Input: part model. Units: mm. Frame: model coordinates. A direction names the side the tool comes from. Coordinates: 2 decimals unless noted, no trailing zeros. Order: outer loops, then holes, each group sorted by start corner. A loop starts at its lowest first (then second) coordinate and runs counter-clockwise, first axis right, second up. Notation, with made-up numbers: (63, -19.75) -> (100, -19.75) arc R21 ccw to (100, 17.25) -> close; hole circle Ø3 at (73, 59). An arc over 180 degrees is marked (long way). Use CSV: the item, a comma, the result in double quotes. Start each with the question number.
Autodesk Inventor part; units mm, degrees
ref_plane "Work Plane1" through (0, 1.5, 0) normal (0, 1, 0) x (1, 0, 0)
ref_plane "YZ Plane" through (0, 0, 0) normal (1, 0, 0) x (0, 1, 0)
ref_plane "XZ Plane" through (0, 0, 0) normal (0, 1, 0) x (-1, 0, 0)
sketch "Sketch1" plane through (0, 0, 0) normal (0, 1, 0) x (-1, 0, 0)
  circle A0 centre (0, 0) radius 8.825
  dimension "d0" = 17.65
extrude "Extrusion1" add sketch "Sketch1" along normal blind 3
sketch "Sketch2" plane through (0, 0, 0) normal (0, -1, 0) x (1, 0, 0)
  circle A0 centre (0, 0) radius 8.825
  circle A1 centre (0, 0) radius 2.75
  dimension "d3" = 5.5
extrude "Extrusion2" add sketch "Sketch2" along normal blind 5 contours A1
sketch "Sketch3" plane through (0, 3, 0) normal (0, 1, 0) x (1, 0, 0)
  circle A0 centre (0, 0) radius 8.825
  circle A1 centre (-6, 0) radius 2
  line L0 (-6, 0) -> (5.0545, 0) construction
  circle A2 centre (0, -6) radius 2
  circle A3 centre (6, 0) radius 2
  circle A4 centre (0, 6) radius 2
  circle A5 centre (-4.2426, 4.2426) radius 0.8
  line L1 (0, 0) -> (-4.2426, 4.2426) construction
  circle A6 centre (0, 0) radius 2.75
  arc A7 (0, 6) -> (-6, 0) centre (0, 0) ccw construction
  circle A8 centre (-4.2426, -4.2426) radius 0.8
  circle A9 centre (4.2426, -4.2426) radius 0.8
  circle A10 centre (4.2426, 4.2426) radius 0.8
  dimension "d6" = 4
  dimension "d7" = 6
  dimension "d10" = 360
  dimension "d14" = 1.6
  dimension "d15" = 45
  dimension "d18" = 360
extrude "Extrusion3" cut sketch "Sketch3" against normal through all contours A1 | A2 | A3 | A4 | A5 | A8 | A9 | A10
sketch "Sketch4" plane through (0, 3, 0) normal (0, 1, 0) x (1, 0, 0)
  circle A0 centre (6, 0) radius 2
  circle A1 centre (-6, 0) radius 2
  circle A2 centre (0, -6) radius 2
  circle A3 centre (0, 6) radius 2
  circle A4 centre (0, 6) radius 2.4
  circle A5 centre (-6, 0) radius 2.4
  circle A6 centre (6, 0) radius 2.4
  circle A7 centre (0, -6) radius 2.4
  dimension "d20" = 0.4
  dimension "d21" = 0.4
  dimension "d22" = 0.4
  dimension "d23" = 0.4
extrude "Extrusion4" cut sketch "Sketch4" against normal blind 0.8
ref_plane "Work Plane1" through (0, 1.5, 0) normal (0, 1, 0) x (1, 0, 0)
mirror "Mirror1" about plane through (0, 1.5, 0) normal (0, 1, 0) of "Extrusion4"
properties part number "xl320_wheel" material "PC/ABS Plastic"
1. Section C-C on x = 6. Return loops of the section in (y, z), then the cut area to 3 significant figures.
2. Contact query for flat-ended pins moving along their axis: P1, Ø1.4, axis at x = 4.24, z = 4.24, coming from the -Y side; P2, Ø2.5, axis at x = -4.24, z = 4.24, coming from the +Y side; P3, Ø5.5, axis at x = 0, z = -7, coming from the -Y side. Output: stop coordinate, or through.
3. Section A-A on z = 0. State how many separate pieces and enclosed holes the cut face has, then the cut area to 3 significant figures.
4. Material intervals for line 1 along Z through (x, y) = (0, 0.55) (3 decimals); line 2 along Z through (x, y) = (-4, 0.25); line 3 along Z through (x, y) = (0.5, 0.25), sorted ascending.
5. Access query for faces 5 (the face through (7, 0.8, -2)), 6 (the face through (-7.6, 1.5, 1.2)), 7 (the face through (-1, 2.2, 4)). Directions: +Z, -Z, +X, -X, +Y, -Y. A direction counts if a zero-diameter tool reaches every point of the face in a straight line with its end or side. Return the directions, or none.
6. Section D-D on y = -1.25. Return loops of the section in (x, z).
7. Pull-direction query (Z, two-part tool) for faces 1 (the face through (0, -5, 0)), 2 (the face through (-0.596, -2.465, 2.685)), 3 (the face through (1.29, 2.606, -8.024)), 4 (the face through (-7, 2.2, -2)); classes: released by +Z, released by -Z, zero draft, split by the parting line, or undercut.
8. Section B-B on z = -7. Return loops of the section in (x, y).
Values follow:
1,outline,"(0, -6.47) -> (3, -6.47) -> (3, -2.4) -> (2.2, -2.4) -> (2.2, -2) -> (0.8, -2) -> (0.8, -2.4) -> (0, -2.4) -> close; (0, 2.4) -> (0.8, 2.4) -> (0.8, 2) -> (2.2, 2) -> (2.2, 2.4) -> (3, 2.4) -> (3, 6.47) -> (0, 6.47) -> close"
1,area,"25.5 mm2"
2,P1,"passes through"
2,P2,"stops at y = 3"
2,P3,"stops at y = 0"
3,separate pieces,"3"
3,enclosed holes,"0"
3,area,"53.9 mm2"
4,line 1,"z = -8.825 to -8.4, -3.6 to 3.6, 8.4 to 8.825"
4,line 2,"z = -7.87 to -5, -3.48 to -1.33, 1.33 to 3.48, 5 to 7.87"
4,line 3,"z = -8.81 to -8.35, -3.65 to 3.65, 8.35 to 8.81"
5,face 5,"-Y"
5,face 6,"+Y, -Y"
5,face 7,"+Y"
6,outline,"circle Ø5.5 at (0, 0)"
7,face 1,"zero draft"
7,face 2,"split by the parting line"
7,face 3,"undercut"
7,face 4,"undercut"
8,outline,"(-5.37, 0) -> (-2.18, 0) -> (-2.18, 0.8) -> (-1.73, 0.8) -> (-1.73, 2.2) -> (-2.18, 2.2) -> (-2.18, 3) -> (-5.37, 3) -> close; (1.73, 0.8) -> (2.18, 0.8) -> (2.18, 0) -> (5.37, 0) -> (5.37, 3) -> (2.18, 3) -> (2.18, 2.2) -> (1.73, 2.2) -> close"
